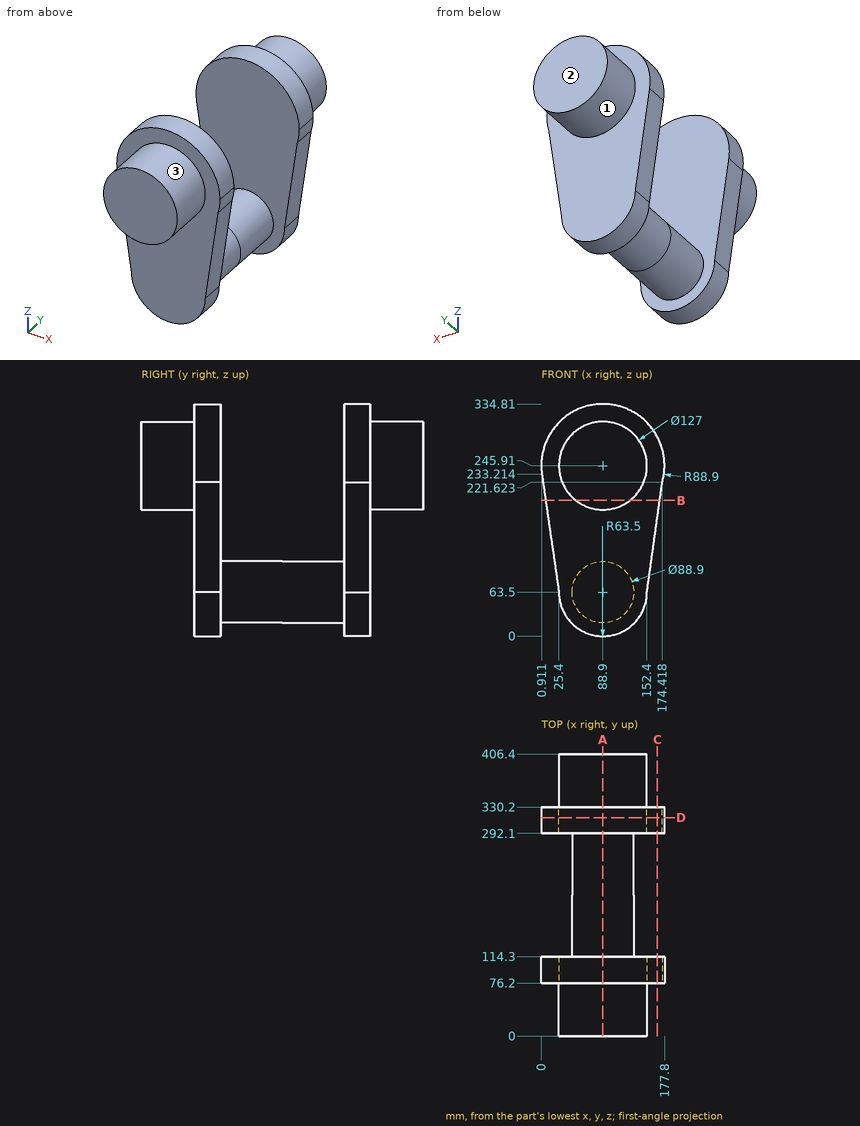
Print and shaded views of the part. All mm, measured from the part's lowest x, y and z. A direction names the side the tool comes from. Round coordinates to 2 decimals unless told otherwise and drop trailing zeros. Write each loop counter-clockwise with the first axis right and the second up, starting at its lowest first coordinate (ties: lowest second). Pieces come first, ordered by that corner, then holes. Notation, with made-up numbers: (-11.75, 54.5) -> (25.25, 54.5) arc R26 ccw to (25.25, 89.5) -> close; hole circle Ø7 at (22.25, -38). An arc over 180 degrees is marked (long way). Return JSON: item names as keys, results as strings. Group by question number.
Q1. Which spindle directions (+Z, -Z, +X, -X, +Y, -Y) get a long thin tool onto all of the face, cutting with end or side? Do the marked faces 1, 2 and 3. Say none if no direction does.
Q2. Pin check, flat tips, straight feed: pin 1 (10 mm diameter, centred on x = 31.5, y = 43, fed in from +Z); pin 2 (1.5 mm diameter, centred on x = 22, z = 136.5, fed in from -Y); pin 3 (1.5 mm diameter, centred on x = 39, z = 81, fed in from +Y). Stop position of each tip, or through.
Q3. Saw through at D-D on y = 315. Write the cut outline in (x, z) (1 decimal), plus the area to 3 significant figures.
Q4. Saw through at C-C on x = 167.5. Write the cut outline in (y, z), plus the area to 3 significant figures.
Q5. Probe L1, parallel to Y at x = 132.5, z = 298.5; L2, parallel to Y at x = 63, z = 57.5; L3, parallel to Z at x = 135.5, y = 292.5 (1 decimal). List the from-to ranges inside material, lowest first. Write a range as [from, to].
Q6. Saw through at B-B on z = 196. Write the cut outline in (x, y), plus the area to 3 significant figures.
Q7. Saw through at A-A on x = 88.9. Write the cut outline in (y, z).
Answer:
{
 "1": {"face 1": "+Y", "face 2": "+Z, -Z, +X, -X, +Y", "face 3": "-Y"},
 "2": {"pin 1": "z = 281.78", "pin 2": "y = 76.2", "pin 3": "y = 330.2"},
 "3": {"outline": "(0.9, 233.2) -> (25.4, 63.5) arc R63.5 ccw to (152.4, 63.5) -> (174.4, 221.6) arc R88.9 ccw to (177.8, 245.9) arc R88.9 ccw (long way) to start", "area": "46,600 mm2"},
 "4": {"outline": "(76.2, 171.94) -> (114.3, 171.94) -> (114.3, 287.45) -> (76.2, 287.45) -> close; (292.1, 171.94) -> (330.2, 171.94) -> (330.2, 287.45) -> (292.1, 287.45) -> close", "area": "8,800 mm2"},
 "5": {"L1": "[76.2, 114.3], [292.1, 330.2]", "L2": "[76.2, 330.2]", "L3": "[20.4, 321.6]"},
 "6": {"outline": "(6.28, 76.2) -> (49.64, 76.2) -> (49.64, 0) -> (128.16, 0) -> (128.16, 76.2) -> (170.85, 76.2) -> (170.85, 114.3) -> (6.28, 114.3) -> close; (6.28, 292.1) -> (170.85, 292.1) -> (170.85, 330.2) -> (128.16, 330.2) -> (128.16, 406.4) -> (49.64, 406.4) -> (49.64, 330.2) -> (6.28, 330.2) -> close", "area": "24,500 mm2"},
 "7": {"outline": "(0, 182.41) -> (76.2, 182.41) -> (76.2, 0) -> (114.3, 0) -> (114.3, 19.05) -> (292.1, 19.05) -> (292.1, 0) -> (330.2, 0) -> (330.2, 182.41) -> (406.4, 182.41) -> (406.4, 309.41) -> (330.2, 309.41) -> (330.2, 334.81) -> (292.1, 334.81) -> (292.1, 107.95) -> (114.3, 107.95) -> (114.3, 334.81) -> (76.2, 334.81) -> (76.2, 309.41) -> (0, 309.41) -> close"}
}
